```python
from build123d import *

# Parameters (mm, degrees)
F1_DEPTH = 63.5
F0_W     = 25.4
F0_H     = 19.05
F0_H_2   = 4.7498
F0_H_3   = 4.7752
F2_DEPTH = 25.4
F4_DEPTH = 3.175
F5_R     = 12.7


with BuildPart() as f1:
    # F0 (on Front) → F1 (new body, symmetric)
    with BuildSketch(Plane.XZ):
        Polygon((-41.275, 9.525), (-41.275, -9.525), (41.275, -9.525), (41.275, 9.525), (22.225, 9.525), align=None)
    extrude(amount=F1_DEPTH, both=True)

    # F0 (on Front) → F2 (join, symmetric)
    with BuildSketch(Plane.XZ):
        with BuildLine():
            Line((22.225, 9.525), (41.275, 9.525))
            Line((41.275, 9.525), (41.275, 27.0002))
            ThreePointArc((41.275, 27.0002), (45.9246798487, 38.2255201513), (57.15, 42.8752))
            Line((57.15, 42.8752), (60.325, 42.8752))
            Line((60.325, 42.8752), (60.325, 61.9252))
            Line((60.325, 61.9252), (57.15, 61.9252))
            add(Edge.make_bspline(
                [(54.8690383613, 61.8506352771), (55.6242381587, 61.8771737888), (56.3845511944, 61.9020277216), (57.15, 61.9252)],
                knots=[110.3049530316, 110.3049530316, 110.3049530316, 110.3049530316, 111.5045361635, 111.5045361635, 111.5045361635, 111.5045361635], degree=3))
            ThreePointArc((54.8690383613, 61.8506352771), (31.6606079885, 50.8758470045), (22.225, 27.0002))
            Line((22.225, 27.0002), (22.225, 9.525))
        make_face()
        with Locations((73.025, 52.4002)):
            Rectangle(F0_W, F0_H)
        with Locations((73.025, 64.3001)):
            Rectangle(F0_W, F0_H_2)
        with Locations((73.025, 40.4876)):
            Rectangle(F0_W, F0_H_3)
    extrude(amount=F2_DEPTH, both=True)

    # F0 (on Front) → F3 (revolve)
    with BuildSketch(Plane.XZ):
        Polygon((85.725, 66.675), (85.725, 61.9252), (85.725, 42.8752), (85.725, 38.1), (111.125, 38.1), (111.125, 66.675), align=None)
    revolve(axis=Axis((85.725, 0, 52.3875), (0, 0, 1)))

    # F0 (on Front) → F4 (join, symmetric)
    with BuildSketch(Plane.XZ):
        with BuildLine():
            add(Edge.make_bspline(
                [(-41.275, 9.525), (-40.782344334, 42.7264267902), (-14.5736504872, 59.4103464678), (54.8690383613, 61.8506352771)],
                knots=[0, 0, 0, 0, 110.3049530316, 110.3049530316, 110.3049530316, 110.3049530316], degree=3))
            Line((-41.275, 9.525), (22.225, 9.525))
            Line((22.225, 9.525), (22.225, 27.0002))
            ThreePointArc((22.225, 27.0002), (31.6606079885, 50.8758470045), (54.8690383613, 61.8506352771))
        make_face()
    extrude(amount=F4_DEPTH, both=True)

    # F5
    f5_edges = [f1.edges().sort_by_distance(p)[0] for p in [
        (85.725, 25.4, 52.3875),
        (73.025, -25.4, 66.675),
        (73.025, 25.4, 66.675),
        (111.125, 0, 66.675),
    ]]
    fillet(f5_edges, radius=F5_R)


solid = f1.part
```
Input: part model. Units: mm. Frame: model coordinates. A direction names the side the tool comes from. Round coordinates to 2 decimals unless told otherwise and drop trailing zeros. Order: outer loops, then holes, each group sorted by start corner. A loop starts at its lowest first (then second) coordinate and runs counter-clockwise, first axis right, second up. Notation, with made-up numbers: (5, 13) - (39, 13) arc R18 ccw to (39, 45) - close; hole circle Ø1 at (78, 41). An arc over 180 degrees is marked (long way). Answer in a Markdown table with one row per item.
Item 1: Section query A-A (y = 55). Return the cut outline in (x, z) (3 decimals).
Model answer:
| item | result |
|---|---|
| outline | (-41.275, -9.525) - (41.275, -9.525) - (41.275, 9.525) - (-41.275, 9.525) - close |
Item 2: Line query: line 1 (X direction, y = -3, z = -2) (3 decimals); line 2 (Z direction, x = 24.5, y = -40) (3 decimals); line 3 (Y direction, x = 61, z = 52). Output: solid intervals per line, ascending.
Model answer:
| item | result |
|---|---|
| line 1 | x = -41.275 to 41.275 |
| line 2 | z = -9.525 to 9.525 |
| line 3 | y = -25.4 to 25.4 |
Item 3: Mould query, pull axis X, two halves, no side actions, for faces 5 (the flat face through (-1, -63.5, 0)), 6 (the flat face through (-41.275, -1, 0)), 7 (the cylindrical face through (45.8, -0.4, 38.1)). Classes: released by +X, released by -X, zero draft, split by the parting line, or undercut.
Model answer:
| item | result |
|---|---|
| face 5 | zero draft |
| face 6 | released by -X |
| face 7 | undercut |
Item 4: Pin query (flat end, axial travel): pin 1 (1 mm diameter, centred on x = 58.5, y = 0.5, fed in from -Z); pin 2 (22 mm diameter, centred on x = 47, z = 41, fed in from -Y); pin 3 (1.5 mm diameter, centred on x = -16, z = 35.5, fed in from +Y) (3 decimals). Return the tip coordinate at first contact, or that it passes through.
Model answer:
| item | result |
|---|---|
| pin 1 | stops at z = 42.88 |
| pin 2 | stops at y = -25.4 |
| pin 3 | stops at y = 3.175 |
Item 5: Reachability of faces 1 (the flat face through (86, 0, 38.1)), 2 (the cylindrical face through (31.91, 14.13, 51.14)), 3 (the flat face through (60.325, 0, 64)), 4 (the flat face through (60.325, 0, 40)) from +Z, -Z, +X, -X, +Y, -Y: full face, straight path, thin tool, end or side. Return the list, or none.
Model answer:
| item | result |
|---|---|
| face 1 | -Z, +X, +Y, -Y |
| face 2 | +Z, -X, +Y |
| face 3 | +Z, -X, +Y, -Y |
| face 4 | -Z, +Y, -Y |
